Read the model definition and answer for the solid it produces. Units are mm, in the model's axes. A direction names the side the tool comes from. Coordinates: 2 decimals unless noted, no trailing zeros. Write each loop counter-clockwise with the first axis right and the second up, starting at its lowest first coordinate (ties: lowest second). Pieces come first, ordered by that corner, then holes.
(1) Which of the six approach directions +Z, -Z, +X, -X, +Y, -Y give full straight-line access (tool end or side, diameter ignored) to faces 5 (the flat face through (91, 116.84, -32)), 6 (the flat face through (91, 247, -38.1))?
(2) The part is cut by section B-B, the plane y = 34. State how many separate pieces and enclosed holes the cut face has, and give its area (3 significant figures).
(3) Determine the mould class of faces 1 (the cylindrical face through (29.22, 123.03, -12.88)), 2 (the cylindrical face through (150.215, 126.986, -12.878)), 3 (the flat face through (184.15, 175, -19)), 4 (the flat face through (91, 142.24, -32)) for opening direction X: pulls with the +X half, pulls with the -X half, needs draft (parallel to the pull), parting line crosses it, or undercut.
(4) Straight lines are drawn through the part: line 1 along Y through (x, z) = (131, -33.5); line 2 along Y through (x, z) = (152.5, -3); line 3 along Z through (x, y) = (22.5, 140.5). For each, find the intervals that lie inside material, in ascending order.
(5) The part is cut by section A-A, the plane y = 129.54. Determine the outline of the cut face in (x, z).
(6) Given pin 1 (3 mm diameter, centred on x = 171.45, z = -19.05, fed in from -Y); pin 2 (14 mm diameter, centred on x = 84, z = -34, fed in from -Y); pin 3 (12.5 mm diameter, centred on x = 77, y = 124.5, fed in from -Z); pin 4 (4 mm diameter, centred on x = 103.41, z = -19.05, fed in from -Y), each flat-ended and moving along its own axis, determine where each tip first touches the part or whether it passes through.
```python
from build123d import *

# Parameters (mm, degrees)
SKETCH1_W                        = 184.15
SKETCH1_H                        = 38.1
BOSS_EXTRUDE1_DEPTH              = 355.6
SKETCH2_W                        = 184.15
SKETCH2_H                        = 25.4
CUT_EXTRUDE1_DEPTH               = 12.7
SKETCH3_R                        = 6.6675
CUT_EXTRUDE2_DEPTH               = 13.7
CUT_EXTRUDE2_DEPTH_BACK          = 26.4
F_10_0_1935_DIAMETER_HOLE1_D     = 4.9149
F_10_0_1935_DIAMETER_HOLE1_DEPTH = 76.2
F_10_0_1935_DIAMETER_HOLE1_TIP   = 1.476584928


with BuildPart() as part:
    # Sketch1 → Boss-Extrude1 (new body)
    with BuildSketch(Plane(origin=(0, 0, 0), x_dir=(1, 0, 0), z_dir=(0, 1, 0))):
        with Locations((92.075, 19.05)):
            Rectangle(SKETCH1_W, SKETCH1_H)
    extrude(amount=BOSS_EXTRUDE1_DEPTH)

    # Sketch2 → Cut-Extrude1 (cut)
    with BuildSketch(Plane.XY.offset(-38.1)):
        with Locations((92.075, 129.54)):
            Rectangle(SKETCH2_W, SKETCH2_H)
    extrude(amount=CUT_EXTRUDE1_DEPTH, mode=Mode.SUBTRACT)

    # Sketch3 → Cut-Extrude2 (cut, two sides)
    with BuildSketch(Plane(origin=(0, 0, -25.4), x_dir=(-1, 0, 0), z_dir=(0, 0, -1))) as cut_extrude2_sk:
        with Locations((-156.37405606, 129.54)):
            Circle(SKETCH3_R)
        with Locations((-27.77594394, 129.54)):
            Circle(SKETCH3_R)
    extrude(amount=CUT_EXTRUDE2_DEPTH, mode=Mode.SUBTRACT)
    extrude(cut_extrude2_sk.sketch, amount=-CUT_EXTRUDE2_DEPTH_BACK, mode=Mode.SUBTRACT)

    # #10 (0.1935) Diameter Hole1
    with Locations(Plane(origin=(12.7, 0, -19.05), x_dir=(0, 0, -1), z_dir=(0, -1, 0))):
        with Locations((0, 0), (0, 22.678571429), (0, 45.357142857), (0, 68.035714286), (0, 90.714285714), (0, 113.392857143), (0, 136.071428571), (0, 158.75)):
            Hole(F_10_0_1935_DIAMETER_HOLE1_D / 2, depth=F_10_0_1935_DIAMETER_HOLE1_DEPTH)
            with Locations((0, 0, -(F_10_0_1935_DIAMETER_HOLE1_DEPTH + F_10_0_1935_DIAMETER_HOLE1_TIP / 2))):  # 118° drill point
                Cone(0, F_10_0_1935_DIAMETER_HOLE1_D / 2, F_10_0_1935_DIAMETER_HOLE1_TIP, mode=Mode.SUBTRACT)


solid = part.part
```
Computed:
1. face 5: -Z, +X, -X
1. face 6: -Z, +X, -X, +Y, -Y
2. separate pieces: 1
2. enclosed holes: 8
2. area: 6,860 mm2
3. face 1: undercut
3. face 2: undercut
3. face 3: pulls with the +X half
3. face 4: needs draft
4. line 1: y = 0 to 116.84, 142.24 to 355.6
4. line 2: y = 0 to 124.11, 134.97 to 355.6
4. line 3: z = -25.4 to 0
5. outline: (0, -25.4) - (21.11, -25.4) - (21.11, 0) - (0, 0) - close; (34.44, -25.4) - (149.71, -25.4) - (149.71, 0) - (34.44, 0) - close; (163.04, -25.4) - (184.15, -25.4) - (184.15, 0) - (163.04, 0) - close
6. pin 1: stops at y = 76.78
6. pin 2: stops at y = 0
6. pin 3: stops at z = -25.4
6. pin 4: stops at y = 76.47
